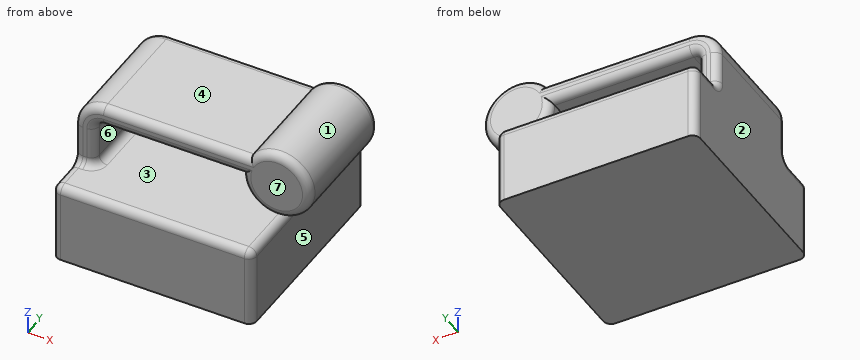
from build123d import *

# Parameters (mm, degrees)
F1_DEPTH = 63.5
F2_DEPTH = 38.1
F3_R     = 5.08


with BuildPart() as f1:
    # F0 (on Front) → F1 (new body, symmetric)
    with BuildSketch(Plane.XZ):
        Polygon((-63.5, 25.4), (-63.5, -25.4), (63.5, -25.4), (63.5, 25.4), (-50.8, 25.4), align=None)
    extrude(amount=F1_DEPTH, both=True)

    # F0 (on Front) → F2 (join, symmetric)
    with BuildSketch(Plane.XZ):
        with BuildLine():
            Line((-63.5, 50.8), (-63.5, 25.4))
            Line((-63.5, 25.4), (-50.8, 25.4))
            Line((-50.8, 25.4), (-50.8, 50.8))
            ThreePointArc((-50.8, 50.8), (-49.1655663717, 54.7458718322), (-45.2196945395, 56.3803054605))
            Line((-45.2196945395, 56.3803054605), (43.2454477532, 56.3803054605))
            ThreePointArc((43.2454477532, 56.3803054605), (44.3071420431, 63.0595111043), (47.3875670326, 69.0803054605))
            Line((47.3875670326, 69.0803054605), (-45.2196945395, 69.0803054605))
            ThreePointArc((-45.2196945395, 69.0803054605), (-58.1458224928, 63.7261279533), (-63.5, 50.8))
        make_face()
        with BuildLine():
            Line((64.7860094905, 69.0803054605), (47.3875670326, 69.0803054605))
            ThreePointArc((47.3875670326, 69.0803054605), (44.3071420431, 63.0595111043), (43.2454477532, 56.3803054605))
            Line((43.2454477532, 56.3803054605), (64.7860094905, 56.3803054605))
            Line((64.7860094905, 56.3803054605), (64.7860094905, 69.0803054605))
        make_face()
        with BuildLine():
            ThreePointArc((86.3265712278, 56.3803054605), (71.4652151342, 76.8591729079), (47.3875670326, 69.0803054605))
            Line((47.3875670326, 69.0803054605), (64.7860094905, 69.0803054605))
            Line((64.7860094905, 69.0803054605), (64.7860094905, 56.3803054605))
            Line((64.7860094905, 56.3803054605), (43.2454477532, 56.3803054605))
            ThreePointArc((43.2454477532, 56.3803054605), (64.7860094905, 34.8397437232), (86.3265712278, 56.3803054605))
        make_face()
    extrude(amount=F2_DEPTH, both=True)

    # F3
    f3_edges = [f1.edges().sort_by_distance(p)[0] for p in [
        (63.5, -63.5, 0),
        (-63.5, -63.5, 0),
        (63.5, 63.5, 0),
        (-63.5, 63.5, 0),
        (-58.145822, -38.1, 63.726128),
        (-63.5, -38.1, 38.1),
        (-57.15, -38.1, 25.4),
        (-50.8, -38.1, 38.1),
        (-49.165566, -38.1, 54.745872),
        (-0.987123, -38.1, 56.380305),
        (85.264877, -38.1, 49.7011),
        (1.083936, -38.1, 69.080305),
        (-58.145822, 38.1, 63.726128),
        (-63.5, 38.1, 38.1),
        (-57.15, 38.1, 25.4),
        (-50.8, 38.1, 38.1),
        (-49.165566, 38.1, 54.745872),
        (-0.987123, 38.1, 56.380305),
        (85.264877, 38.1, 49.7011),
        (1.083936, 38.1, 69.080305),
        (0, -63.5, 25.4),
        (63.5, 0, 25.4),
        (0, 63.5, 25.4),
        (-63.5, -50.8, 25.4),
        (-63.5, 50.8, 25.4),
        (-50.8, 0, 25.4),
    ]]
    fillet(f3_edges, radius=F3_R)


solid = f1.part
Geometry: final body of the model. Coordinates: model frame, mm. Face numbers are marked on the shaded views. A direction names the side the tool comes from. Coordinates: 2 decimals unless noted, no trailing zeros. Order: outer loops, then holes, each group sorted by start corner. A loop starts at its lowest first (then second) coordinate and runs counter-clockwise, first axis right, second up.
(1) Material intervals for probe 1 along Z at (x, y) = (-25, -4); probe 2 along Z at (x, y) = (51, -41); probe 3 along X at (y, z) = (-52.5, 1.5), sorted ascending.
(2) Draft query along X for the marked faces 1, 2 and 3. Return one class per face: pulls with the +X half, pulls with the -X half, needs draft (parallel to the pull), parting line crosses it, or undercut.
(3) First-contact query: pin 1 (12 mm diameter, centred on x = 62.5, y = -47, fed in from +Z); pin 2 (10 mm diameter, centred on y = -1, z = 44, fed in from +X); pin 3 (4 mm diameter, centred on y = 4, z = -0.5, fed in from +X). Flat tips, straight axial feed; report the tip coordinate or a pass-through.
(4) Section query B-B (y = 18.5). Return the cut outline in (x, z), plus the area to 3 significant figures.
(5) Access query for the marked faces 4, 5, 6 and 7. Directions: +Z, -Z, +X, -X, +Y, -Y. A direction counts if a zero-diameter tool reaches every point of the face in a straight line with its end or side. Return the directions, or none.
(6) Section query A-A (x = 16.5). Return the cut outline in (y, z), plus the area to 3 significant figures.
(7) Section query C-C (z = -5). Return the cut outline in (x, y), plus the area to 3 significant figures.
Solution:
1. probe 1: z = -25.4 to 25.4, 56.38 to 69.08
1. probe 2: z = -25.4 to 25.4
1. probe 3: x = -63.5 to 63.5
2. face 1: undercut
2. face 2: pulls with the -X half
2. face 3: needs draft
3. pin 1: stops at z = 25.4
3. pin 2: stops at x = 85.02
3. pin 3: stops at x = 63.5
4. outline: (-63.5, -25.4) - (63.5, -25.4) - (63.5, 20.32) arc R5.08 ccw to (58.42, 25.4) - (-45.72, 25.4) arc R5.08 cw to (-50.8, 30.48) - (-50.8, 50.8) arc R5.58 cw to (-45.22, 56.38) - (43.25, 56.38) arc R21.54 ccw (long way) to (47.39, 69.08) - (-45.22, 69.08) arc R18.28 ccw to (-63.5, 50.8) - close
4. area: 9,610 mm2
5. face 4: +Z, -X, +Y, -Y
5. face 5: -Z, +X, +Y, -Y
5. face 6: +Y, -Y
5. face 7: +Z, +X, -X, -Y
6. outline: (-63.5, -25.4) - (63.5, -25.4) - (63.5, 20.32) arc R5.08 ccw to (58.42, 25.4) - (-58.42, 25.4) arc R5.08 ccw to (-63.5, 20.32) - close; (-38.1, 61.46) arc R5.08 ccw to (-33.02, 56.38) - (33.02, 56.38) arc R5.08 ccw to (38.1, 61.46) - (38.1, 64) arc R5.08 ccw to (33.02, 69.08) - (-33.02, 69.08) arc R5.08 ccw to (-38.1, 64) - close
6. area: 7,390 mm2
7. outline: (-63.5, -58.42) arc R5.08 ccw to (-58.42, -63.5) - (58.42, -63.5) arc R5.08 ccw to (63.5, -58.42) - (63.5, 58.42) arc R5.08 ccw to (58.42, 63.5) - (-58.42, 63.5) arc R5.08 ccw to (-63.5, 58.42) - close
7. area: 16,100 mm2
